Input: part model. Units: mm. Frame: model coordinates. A direction names the side the tool comes from. Round coordinates to 2 decimals unless told otherwise and drop trailing zeros. Loops run counter-clockwise (first coordinate to the right, second up) from the corner with the lowest first, then second, coordinate; pieces in that order, holes last.
(1) First-contact query: pin 1 Ø5.5 at (x, y) = (-52.5, -122.5) entering from -Z; pin 2 Ø1.8 at (x, z) = (40.5, 17.42) entering from -Y; pin 3 Ø1.8 at (x, z) = (-11.78, 82.47) entering from +Y; pin 4 Ø2.5 at (x, z) = (34.76, 69.22) entering from -Y. Flat tips, straight axial feed; report the tip coordinate or a pass-through.
(2) Cut plane A-A, the plane y = -99. Output: boundary loops of the cut face in (x, z), and give its area (3 significant figures).
(3) Cut plane C-C, the plane z = 92.5. Output: boundary loops of the cut face in (x, y), and give its area (3 significant figures).
(4) Cut plane D-D, the plane x = 0.5. Output: boundary loops of the cut face in (y, z), and give its area (3 significant figures).
(5) Draft query along X for faces 6 (the face through (66.558, -122, 50)), 7 (the face through (22, 118.1, 49)), 8 (the face through (100, -2, 49)), 9 (the face through (-97, 113.272, 50)). Return one class per face: released by +X, released by -X, zero draft, split by the parting line, or undercut.
(6) Line query: line 1 (X direction, y = -70.5, z = 40); line 2 (Y direction, x = 50, z = 18); line 3 (Y direction, x = 51, z = 55.5). Output: solid intervals per line, ascending.
(7) Cut plane B-B, the plane x = -84. Output: boundary loops of the cut face in (y, z).
(8) Access query for faces 1 (the face through (0, 122, 20.17)), 2 (the face through (-97, 83, 64.818)), 3 (the face through (1, -118.1, 49)), 4 (the face through (-97, 1, 100)), 5 (the face through (-52, -122, 79.723)). Directions: +Z, -Z, +X, -X, +Y, -Y. A direction counts if a zero-diameter tool reaches every point of the face in a straight line with its end or side. Return the directions, or none.
from build123d import *

# Parameters (mm, degrees)
ESBO_O1_W                  = 200
ESBO_O1_H                  = 250
RESSALTO_EXTRUS_O2_DEPTH   = 100
ESBO_O6_W                  = 186.2
ESBO_O6_H                  = 236.2
CORTE_EXTRUS_O3_DEPTH      = 100
ESBO_O7_W                  = 29
ESBO_O7_H                  = 59.5
CORTE_EXTRUS_O4_DEPTH      = 213
FILETE1_R                  = 3
CORTE_EXTRUS_O6_DEPTH      = 189.745860882
CORTE_EXTRUS_O6_DEPTH_BACK = 189.745860882
ESBO_O8_R                  = 1.025
CHANFRO2_SIZE              = 0.325
CHANFRO3_SIZE              = 0.325
ESBO_O10_W                 = 29.5
ESBO_O10_H                 = 59.5
CORTE_EXTRUS_O7_DEPTH      = 47
FILETE2_R                  = 3
ESBO_O11_R                 = 1.025
CORTE_EXTRUS_O8_DEPTH      = 9
CHANFRO4_SIZE              = 0.325
ESBO_O12_W                 = 29
ESBO_O12_H                 = 59.5
CORTE_EXTRUS_O9_DEPTH      = 23
FILETE3_R                  = 3
ESBO_O13_R                 = 1.025
CORTE_EXTRUS_O10_DEPTH     = 23
CHANFRO5_SIZE              = 0.325


with BuildPart() as part:
    # Esboço1 → Ressalto-extrusão2 (new body)
    with BuildSketch(Plane.XY):
        Rectangle(ESBO_O1_W, ESBO_O1_H)
    extrude(amount=RESSALTO_EXTRUS_O2_DEPTH)

    # Esboço6 → Corte-extrusão3 (cut)
    with BuildSketch(Plane(origin=(0, 0, 0), x_dir=(-1, 0, 0), z_dir=(0, 0, -1))):
        Rectangle(ESBO_O6_W, ESBO_O6_H)
    extrude(amount=-CORTE_EXTRUS_O3_DEPTH, mode=Mode.SUBTRACT)

    # Esboço7 → Corte-extrusão4 (cut)
    with BuildSketch(Plane(origin=(100, 0, 0), x_dir=(0, 0, -1), z_dir=(1, 0, 0))):
        with Locations((-50.318421244, 83.522264674)):
            Rectangle(ESBO_O7_W, ESBO_O7_H)
    extrude(amount=-CORTE_EXTRUS_O4_DEPTH, mode=Mode.SUBTRACT)

    # Filete1
    filete1_edges = [part.edges().sort_by_distance(p)[0] for p in [
        (-96.55, 53.772264674, 64.818421244),
        (96.55, 53.772264674, 64.818421244),
        (-96.55, 113.272264674, 64.818421244),
        (96.55, 113.272264674, 64.818421244),
        (-96.55, 113.272264674, 35.818421244),
        (96.55, 113.272264674, 35.818421244),
        (-96.55, 53.772264674, 35.818421244),
        (96.55, 53.772264674, 35.818421244),
    ]]
    fillet(filete1_edges, radius=FILETE1_R)

    # Esboço8 → Corte-extrusão6 (cut, two sides: drawn at the far end of the back side and taken through both)
    with BuildSketch(Plane(origin=(0, 0, 0), x_dir=(0, 0, -1), z_dir=(1, 0, 0)).offset(-CORTE_EXTRUS_O6_DEPTH_BACK)):
        with Locations((-67.618421244, 102.772264674)):
            Circle(ESBO_O8_R)
        with Locations((-67.618421244, 80.772264674)):
            Circle(ESBO_O8_R)
        with Locations((-67.618421244, 58.772264674)):
            Circle(ESBO_O8_R)
        with Locations((-61.818421244, 50.972264674)):
            Circle(ESBO_O8_R)
        with Locations(Location((-38.818421244, 50.972264674, 0), (0, 0, 270))):
            Circle(ESBO_O8_R)
        with Locations(Location((-33.018421244, 58.772264674, 0), (0, 0, 270))):
            Circle(ESBO_O8_R)
        with Locations(Location((-33.018421244, 80.772264674, 0), (0, 0, 270))):
            Circle(ESBO_O8_R)
        with Locations(Location((-33.018421244, 102.772264674, 0), (0, 0, 270))):
            Circle(ESBO_O8_R)
    extrude(amount=CORTE_EXTRUS_O6_DEPTH + CORTE_EXTRUS_O6_DEPTH_BACK, mode=Mode.SUBTRACT)

    # Chanfro2
    chanfro2_edges = [part.edges().sort_by_distance(p)[0] for p in [
        (100, 103.797264674, 33.018421244),
        (100, 81.797264674, 33.018421244),
        (100, 59.797264674, 33.018421244),
        (100, 51.997264674, 38.818421244),
        (100, 50.972264674, 62.843421244),
        (100, 58.772264674, 68.643421244),
        (100, 80.772264674, 68.643421244),
        (100, 102.772264674, 68.643421244),
    ]]
    chamfer(chanfro2_edges, length=CHANFRO2_SIZE)

    # Chanfro3
    chanfro3_edges = [part.edges().sort_by_distance(p)[0] for p in [
        (-100, 103.797264674, 33.018421244),
        (-100, 81.797264674, 33.018421244),
        (-100, 59.797264674, 33.018421244),
        (-100, 51.997264674, 38.818421244),
        (-100, 50.972264674, 62.843421244),
        (-100, 58.772264674, 68.643421244),
        (-100, 80.772264674, 68.643421244),
        (-100, 102.772264674, 68.643421244),
    ]]
    chamfer(chanfro3_edges, length=CHANFRO3_SIZE)

    # Esboço10 → Corte-extrusão7 (cut)
    with BuildSketch(Plane(origin=(0, 125, 0), x_dir=(1, 0, 0), z_dir=(0, 1, 0))):
        with Locations((-0.032057976, -49.919885363)):
            Rectangle(ESBO_O10_W, ESBO_O10_H)
    extrude(amount=-CORTE_EXTRUS_O7_DEPTH, mode=Mode.SUBTRACT)

    # Filete2
    filete2_edges = [part.edges().sort_by_distance(p)[0] for p in [
        (-14.782057976, 121.55, 79.669885363),
        (-14.782057976, 121.55, 20.169885363),
        (14.717942024, 121.55, 20.169885363),
        (14.717942024, 121.55, 79.669885363),
    ]]
    fillet(filete2_edges, radius=FILETE2_R)

    # Esboço11 → Corte-extrusão8 (cut)
    with BuildSketch(Plane(origin=(0, 125, 0), x_dir=(1, 0, 0), z_dir=(0, 1, 0))):
        with Locations(Location((-17.582057976, -30.669885363, 0), (0, 0, 180))):
            Circle(ESBO_O11_R)
        with Locations(Location((-17.582057976, -52.669885363, 0), (0, 0, 180))):
            Circle(ESBO_O11_R)
        with Locations(Location((-17.582057976, -74.669885363, 0), (0, 0, 180))):
            Circle(ESBO_O11_R)
        with Locations(Location((-11.782057976, -82.469885363, 0), (0, 0, 180))):
            Circle(ESBO_O11_R)
        with Locations(Location((11.717942024, -82.469885363, 0), (0, 0, 180))):
            Circle(ESBO_O11_R)
        with Locations(Location((17.517942024, -74.669885363, 0), (0, 0, 180))):
            Circle(ESBO_O11_R)
        with Locations(Location((17.517942024, -52.669885363, 0), (0, 0, 180))):
            Circle(ESBO_O11_R)
        with Locations(Location((17.517942024, -30.669885363, 0), (0, 0, 180))):
            Circle(ESBO_O11_R)
    extrude(amount=-CORTE_EXTRUS_O8_DEPTH, mode=Mode.SUBTRACT)

    # Chanfro4
    chanfro4_edges = [part.edges().sort_by_distance(p)[0] for p in [
        (18.542942024, 125, 30.669885363),
        (18.542942024, 125, 52.669885363),
        (18.542942024, 125, 74.669885363),
        (12.742942024, 125, 82.469885363),
        (-10.757057976, 125, 82.469885363),
        (-16.557057976, 125, 74.669885363),
        (-16.557057976, 125, 52.669885363),
        (-16.557057976, 125, 30.669885363),
    ]]
    chamfer(chanfro4_edges, length=CHANFRO4_SIZE)

    # Esboço12 → Corte-extrusão9 (cut)
    with BuildSketch(Plane.XZ.offset(125)):
        with Locations((52.057675452, 49.972658861)):
            Rectangle(ESBO_O12_W, ESBO_O12_H)
        with Locations((-52.057675452, 49.972658861)):
            Rectangle(ESBO_O12_W, ESBO_O12_H)
    extrude(amount=-CORTE_EXTRUS_O9_DEPTH, mode=Mode.SUBTRACT)

    # Filete3
    filete3_edges = [part.edges().sort_by_distance(p)[0] for p in [
        (-66.557675452, -121.55, 20.222658861),
        (-66.557675452, -121.55, 79.722658861),
        (-37.557675452, -121.55, 79.722658861),
        (-37.557675452, -121.55, 20.222658861),
        (37.557675452, -121.55, 20.222658861),
        (37.557675452, -121.55, 79.722658861),
        (66.557675452, -121.55, 79.722658861),
        (66.557675452, -121.55, 20.222658861),
    ]]
    fillet(filete3_edges, radius=FILETE3_R)

    # Esboço13 → Corte-extrusão10 (cut)
    with BuildSketch(Plane.XZ.offset(125)):
        with Locations((-69.357675452, 69.222658861)):
            Circle(ESBO_O13_R)
        with Locations((-69.357675452, 47.222658861)):
            Circle(ESBO_O13_R)
        with Locations((-69.357675452, 25.222658861)):
            Circle(ESBO_O13_R)
        with Locations((-63.610686645, 17.422658861)):
            Circle(ESBO_O13_R)
        with Locations((-40.50466426, 17.422658861)):
            Circle(ESBO_O13_R)
        with Locations((-34.757675452, 25.222658861)):
            Circle(ESBO_O13_R)
        with Locations((-34.757675452, 47.222658861)):
            Circle(ESBO_O13_R)
        with Locations((-34.757675452, 69.222658861)):
            Circle(ESBO_O13_R)
        with Locations((34.757675452, 25.222658861)):
            Circle(ESBO_O13_R)
        with Locations((40.50466426, 17.422658861)):
            Circle(ESBO_O13_R)
        with Locations((63.610686645, 17.422658861)):
            Circle(ESBO_O13_R)
        with Locations((69.357675452, 25.222658861)):
            Circle(ESBO_O13_R)
        with Locations((69.357675452, 47.222658861)):
            Circle(ESBO_O13_R)
        with Locations((34.757675452, 47.222658861)):
            Circle(ESBO_O13_R)
        with Locations((34.757675452, 69.222658861)):
            Circle(ESBO_O13_R)
        with Locations((69.357675452, 69.222658861)):
            Circle(ESBO_O13_R)
    extrude(amount=-CORTE_EXTRUS_O10_DEPTH, mode=Mode.SUBTRACT)

    # Chanfro5
    chanfro5_edges = [part.edges().sort_by_distance(p)[0] for p in [
        (-35.782675452, -125, 47.222658861),
        (-35.782675452, -125, 25.222658861),
        (-41.52966426, -125, 17.422658861),
        (-64.635686645, -125, 17.422658861),
        (39.47966426, -125, 17.422658861),
        (-70.382675452, -125, 69.222658861),
        (-70.382675452, -125, 47.222658861),
        (-70.382675452, -125, 25.222658861),
        (68.332675452, -125, 69.222658861),
        (33.732675452, -125, 69.222658861),
        (33.732675452, -125, 47.222658861),
        (68.332675452, -125, 47.222658861),
        (68.332675452, -125, 25.222658861),
        (62.585686645, -125, 17.422658861),
        (-35.782675452, -125, 69.222658861),
        (33.732675452, -125, 25.222658861),
    ]]
    chamfer(chanfro5_edges, length=CHANFRO5_SIZE)


solid = part.part
Reported:
1. pin 1: stops at z = 0
1. pin 2: stops at y = 118.1
1. pin 3: stops at y = -118.1
1. pin 4: stops at y = -124.9
2. outline: (-100, 0) - (-93.1, 0) - (-93.1, 100) - (-100, 100) - close; (93.1, 0) - (100, 0) - (100, 100) - (93.1, 100) - close
2. area: 1,380 mm2
3. outline: (-100, -125) - (100, -125) - (100, 125) - (-100, 125) - close; hole (-93.1, -118.1) - (93.1, -118.1) - (93.1, 118.1) - (-93.1, 118.1) - close
3. area: 6,020 mm2
4. outline: (-125, 0) - (-118.1, 0) - (-118.1, 100) - (-125, 100) - close; (118.1, 0) - (125, 0) - (125, 20.17) - (118.1, 20.17) - close; (118.1, 79.67) - (125, 79.67) - (125, 100) - (118.1, 100) - close
4. area: 969 mm2
5. face 6: undercut
5. face 7: undercut
5. face 8: released by +X
5. face 9: zero draft
6. line 1: x = -100 to -93.1, 93.1 to 100
6. line 2: y = -125 to -118.1, 118.1 to 125
6. line 3: y = 118.1 to 125
7. outline: (-125, 0) - (-118.1, 0) - (-118.1, 100) - (-125, 100) - close; (118.1, 0) - (125, 0) - (125, 100) - (118.1, 100) - close
8. face 1: +Y
8. face 2: +X, -X
8. face 3: +Z, -Z
8. face 4: +Z, +X, -X, +Y, -Y
8. face 5: -Y
